Autodesk Inventor part; units mm, degrees
ref_plane "YZ Plane" through (0, 0, 0) normal (1, 0, 0) x (0, 1, 0)
ref_plane "XZ Plane" through (0, 0, 0) normal (0, 1, 0) x (-1, 0, 0)
ref_plane "XY Plane" through (0, 0, 0) normal (0, 0, 1) x (1, 0, 0)
sketch "Sketch1" plane through (0, 0, 0) normal (0, 1, 0) x (-1, 0, 0)
  circle A0 centre (0, 0) radius 6.5
  dimension "d0" = 13
extrude "Extrusion1" add sketch "Sketch1" along normal blind 109
chamfer "Chamfer1" distance 3 angle 45 1 edges at (6.5, 0, 0)
sketch "Sketch2" plane through (0, 0, 0) normal (1, 0, 0) x (0, 1, 0)
  line L0 (20, 11.2856) -> (-12.0513, 11.2856)
  line L1 (-12.0513, 11.2856) -> (-12.0513, -8.7625)
  line L2 (-12.0513, -8.7625) -> (20, -8.7625)
  line L3 (20, -8.7625) -> (20, 11.2856)
  line L4 (109, -6.5) -> (109, 6.5) construction
  line L5 (3, 6.5) -> (3, -6.5) construction
  line L6 (0, -3.5) -> (0, 3.5) construction
  point P0 (0, 0)
  dimension "d6" = 20
extrude "Extrusion2" cut sketch "Sketch2" along normal mid plane 3
sketch "Sketch3" plane through (0, 0, 0) normal (1, 0, 0) x (0, 1, 0)
  line L0 (-21.8, 0) -> (130.8, 0) construction
  line L1 (0, -3.1623) -> (0, 3.1623) construction
  point P0 (0, 0)
  point P1 (10, 0)
  dimension "d9" = 10
hole "Hole1" at (0, 10, 0) direction (1, 0, 0) diameter 3 end through all
mirror "Mirror1" about plane through (0, 0, 0) normal (1, 0, 0) of "Hole1"
properties part number "LIVER SHAFT" material "Steel, Alloy"
Verification items for the finished model (mm, model axes). A direction names the side the tool comes from. Give positions to 0.01 mm unless a question says otherwise; leave off trailing zeros. Order: outer loops, then holes, each group sorted by start corner. A loop starts at its lowest first (then second) coordinate and runs counter-clockwise, first axis right, second up. Notation, with made-up numbers: (72.25, -13) -> (118.25, -13) arc R22 cw to (118.25, 1) -> close; hole circle Ø3 at (-4, 46.5). An arc over 180 degrees is marked (long way). Answer as CSV lines item,"result".
Q1. Sectioned sample at C-C on x = 0. Record the cut outline in (y, z).
Solutions:
outline,"(20, -6.5) -> (109, -6.5) -> (109, 6.5) -> (20, 6.5) -> close"
Q2. Sectioned sample at A-A on y = 10. Record the cut outline in (x, z), plus the area to 3 significant figures.
Solutions:
outline,"(-6.32, -1.5) arc R6.5 ccw to (-1.5, -6.32) -> (-1.5, -1.5) -> close; (-6.32, 1.5) -> (-1.5, 1.5) -> (-1.5, 6.32) arc R6.5 ccw to start; (1.5, -6.32) arc R6.5 ccw to (6.32, -1.5) -> (1.5, -1.5) -> close; (1.5, 1.5) -> (6.32, 1.5) arc R6.5 ccw to (1.5, 6.32) -> close"
area,"64.4 mm²"
Q3. Sectioned sample at B-B on z = 0. Record the cut outline in (x, y).
Solutions:
outline,"(-6.5, 3) -> (-3.5, 0) -> (-1.5, 0) -> (-1.5, 8.5) -> (-6.5, 8.5) -> close; (-6.5, 11.5) -> (-1.5, 11.5) -> (-1.5, 20) -> (1.5, 20) -> (1.5, 11.5) -> (6.5, 11.5) -> (6.5, 109) -> (-6.5, 109) -> close; (1.5, 0) -> (3.5, 0) -> (6.5, 3) -> (6.5, 8.5) -> (1.5, 8.5) -> close"
Q4. Release check for a two-part mould opening along X. For faces 3 (the conical face through (-4.4, 0.9, -0.1)), 4 (the cylindrical face through (4.035, 11.464, -0.325)), 5 (the cylindrical face through (-6.2, 55.26, -1.95)), 6 (the flat face through (0, 20, 0)) record: +X half, -X half, draft (parallel to the pull), parting line (faces both ways), or undercut.
Solutions:
face 3,"-X half"
face 4,"draft"
face 5,"parting line"
face 6,"undercut"
Q5. Sectioned sample at D-D on y = 28.5. Record the cut outline in (x, z), plus the area to 3 significant figures.
Solutions:
outline,"circle Ø13 at (0, 0)"
area,"133 mm²"
Q6. Scan lines: probe 1 along Y at (x, z) = (3.35, 0); probe 2 along X at (y, z) = (11.5, -3.25); probe 3 along Y at (x, z) = (1.25, 1). Record each from-to range of solid material in increasing order.
Solutions:
probe 1,"y = 0 to 8.5, 11.5 to 109"
probe 2,"x = -5.63 to -1.5, 1.5 to 5.63"
probe 3,"y = 20 to 109"
Q7. Access from +Z, -Z, +X, -X, +Y, -Y to the whole of each face (thin tool, end or side, straight path). Record for faces 1 (the flat face through (1.5, 12, 0)), 2 (the flat face through (0, 109, 0)).
Solutions:
face 1,"+Z, -Z, -Y"
face 2,"+Z, -Z, +X, -X, +Y"
Q8. Depth check by flat-ended pin: pin 1 (0.9 mm diameter, centred on x = 0, z = 3, fed in from -Y); pin 2 (6 mm diameter, centred on x = 2.5, y = 13, fed in from -Z); pin 3 (1.8 mm diameter, centred on y = 10, z = 0, fed in from -X); pin 4 (1.5 mm diameter, centred on x = -3, y = 39.5, fed in from -Z). Enter the tip coordinate at first touch or a pass-through.
Solutions:
pin 1,"stops at y = 20"
pin 2,"stops at z = -6.32"
pin 3,"passes through"
pin 4,"stops at z = -6.1"
